Work out the finished part from the listing and answer in its coordinate system (mm). Face numbers are marked on the shaded views. A direction names the side the tool comes from. Round coordinates to 2 decimals unless told otherwise and drop trailing zeros. Loops run counter-clockwise (first coordinate to the right, second up) from the corner with the lowest first, then second, coordinate; pieces in that order, holes last. Notation, with made-up numbers: (75.5, 77.25) - (115.5, 77.25) arc R13 cw to (115.5, 99.25) - close; hole circle Ø2 at (58.25, 27.5). An arc over 180 degrees is marked (long way). Use CSV: the item, a comma, the result in double quotes. Start each with the question number.
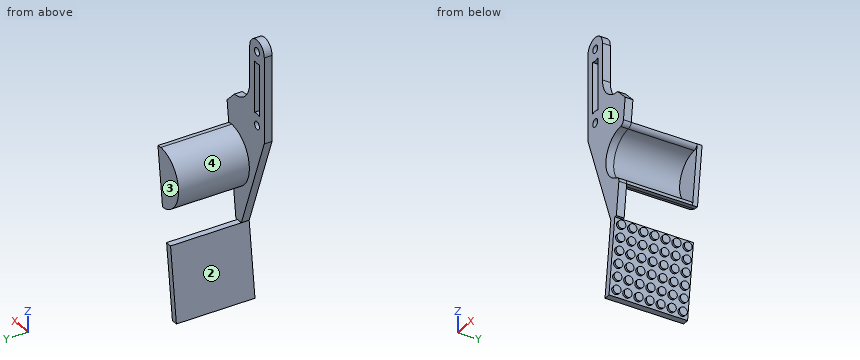
from build123d import *
from build123d.topology import SkipClean

# Parameters (mm, degrees)
CROQUIS1_R              = 1.5875
SALIENTE_EXTRUIR1_DEPTH = 3.175
CORTAR_EXTRUIR1_DEPTH   = 3.175
CORTAR_EXTRUIR3_DEPTH   = 10
CROQUIS4_R              = 10
CORTAR_EXTRUIR4_DEPTH   = 10
REDONDEO1_R             = 2
BOSS_EXTRUDE1_DEPTH     = 26.82
BOSS_EXTRUDE2_DEPTH     = 2
BOSS_EXTRUDE3_DEPTH     = 31.995
SKETCH5_R               = 1.59
BOSS_EXTRUDE4_DEPTH     = 1


with BuildPart() as part:
    # Croquis1 → Saliente-Extruir1 (new body)
    with BuildSketch(Plane(origin=(0, 0, 0), x_dir=(1, 0, 0), z_dir=(0, 1, 0))):
        with BuildLine():
            Line((-12.5, 0), (-12.5, -40))
            Line((-12.5, -40), (-2.975, -40))
            Line((-2.975, -40), (-2.975, -20))
            ThreePointArc((-2.975, -20), (-0.046067812, -12.928932188), (7.025, -10))
            Line((7.025, -10), (12.5, -10))
            Line((12.5, -10), (12.5, 40))
            Line((12.5, 40), (2.5, 40))
            Line((2.5, 40), (-12.5, 0))
        make_face()
        with Locations(Location((-7.7375, -5, 0), (0, 0, 270))):
            Circle(CROQUIS1_R, mode=Mode.SUBTRACT)
        with Locations(Location((-7.7375, -35, 0), (0, 0, 270))):
            Circle(CROQUIS1_R, mode=Mode.SUBTRACT)
    extrude(amount=SALIENTE_EXTRUIR1_DEPTH)

    # Croquis2 → Cortar-Extruir1 (cut)
    with BuildSketch(Plane(origin=(0, 3.175, 0), x_dir=(1, 0, 0), z_dir=(0, 1, 0))):
        Polygon((12.5, -10), (6.1, 40), (12.5, 40), align=None)
    extrude(amount=-CORTAR_EXTRUIR1_DEPTH, mode=Mode.SUBTRACT)

    # Croquis3 → Cortar-Extruir3 (cut)
    with BuildSketch(Plane(origin=(0, 3.175, 0), x_dir=(1, 0, 0), z_dir=(0, 1, 0))):
        with BuildLine():
            ThreePointArc((-5.975, -30.575635639), (-7.7375, -30.2375), (-9.5, -30.575635639))
            Line((-9.5, -30.575635639), (-9.5, -9.427055314))
            ThreePointArc((-9.5, -9.427055314), (-7.7375, -9.765), (-5.975, -9.427055314))
            Line((-5.975, -9.427055314), (-5.975, -14.803847577))
            Line((-5.975, -14.803847577), (-5.975, -30.575635639))
        make_face()
        with BuildLine():
            ThreePointArc((-12.5, -35), (-7.7375, -39.7625), (-2.975, -35))
            Line((-2.975, -35), (-2.975, -40))
            Line((-2.975, -40), (-12.5, -40))
            Line((-12.5, -40), (-12.5, -35))
        make_face()
    extrude(amount=-CORTAR_EXTRUIR3_DEPTH, mode=Mode.SUBTRACT)

    # Croquis4 → Cortar-Extruir4 (cut)
    with BuildSketch(Plane(origin=(0, 3.175, 0), x_dir=(1, 0, 0), z_dir=(0, 1, 0))):
        with Locations((9.274103387, 15.202317292)):
            Circle(CROQUIS4_R)
        Polygon((7.025, -10), (11.878723404, -5.146276596), (12.5, -10), align=None)
    extrude(amount=-CORTAR_EXTRUIR4_DEPTH, mode=Mode.SUBTRACT)

    # Redondeo1
    redondeo1_edges = [part.edges().sort_by_distance(p)[0] for p in [
        (8.004462032, 1.5875, -25.121390375),
        (10.543744741, 1.5875, -5.283244209),
    ]]
    fillet(redondeo1_edges, radius=REDONDEO1_R)

    # Sketch1 → Boss-Extrude1 (add)
    with SkipClean():  # the faces are left unmerged after this step: merging them gives an invalid solid
        with BuildSketch(Plane(origin=(0, 3.175, 0), x_dir=(1, 0, 0), z_dir=(0, 1, 0))):
            with BuildLine():
                Line((7.771843477, 26.938722839), (5.78802886, 26.684794568))
                ThreePointArc((5.78802886, 26.684794568), (-2.628784313, 13.678747666), (8.79254868, 3.211983474))
                Line((8.79254868, 3.211983474), (10.776363297, 3.465911745))
                ThreePointArc((10.776363297, 3.465911745), (10.143802127, 4.686471223), (8.872807798, 5.210372444))
                ThreePointArc((8.872807798, 5.210372444), (-0.644969697, 13.932675937), (6.369041281, 24.771048355))
                ThreePointArc((6.369041281, 24.771048355), (7.467102295, 25.59818866), (7.771843477, 26.938722839))
            make_face()
        extrude(amount=BOSS_EXTRUDE1_DEPTH)

    # Sketch2 → Boss-Extrude2 (add)
    with SkipClean():  # the faces are left unmerged after this step: merging them gives an invalid solid
        with BuildSketch(Plane(origin=(0, 29.995, 0), x_dir=(1, 0, 0), z_dir=(0, 1, 0))):
            with BuildLine():
                Line((10.776363297, 3.465911745), (7.771843477, 26.938722839))
                Line((7.771843477, 26.938722839), (5.78802886, 26.684794568))
                ThreePointArc((5.78802886, 26.684794568), (-2.628784313, 13.678747666), (8.79254868, 3.211983474))
                Line((8.79254868, 3.211983474), (10.776363297, 3.465911745))
            make_face()
        extrude(amount=BOSS_EXTRUDE2_DEPTH)

    # Sketch4 → Boss-Extrude3 (add)
    with SkipClean():  # the faces are left unmerged after this step: merging them gives an invalid solid
        with BuildSketch(Plane.XZ):
            Polygon((1.291075936, -69.75721925), (-1.308924064, -69.75721925), (2.5, -40), (5.1, -40), align=None)
        extrude(amount=-BOSS_EXTRUDE3_DEPTH)

    # Sketch5 → Boss-Extrude4 (add)
    with SkipClean():  # the faces are left unmerged after this step: merging them gives an invalid solid
        with BuildSketch(Plane(origin=(10.055254707, 0, -1.287072602), x_dir=(-0.12696413546540494, 0, -0.9919073083234755), z_dir=(0.9919073083234755, 0, -0.12696413546540494))):
            with Locations((41.528775242, 29.495)):
                Circle(SKETCH5_R)
            with Locations((46.528775242, 29.495)):
                Circle(SKETCH5_R)
            with Locations((51.528775242, 29.495)):
                Circle(SKETCH5_R)
            with Locations((56.528775242, 29.495)):
                Circle(SKETCH5_R)
            with Locations((61.528775242, 29.495)):
                Circle(SKETCH5_R)
            with Locations((66.528775242, 29.495)):
                Circle(SKETCH5_R)
            with Locations((46.528775242, 24.995)):
                Circle(SKETCH5_R)
            with Locations((51.528775242, 24.995)):
                Circle(SKETCH5_R)
            with Locations((56.528775242, 24.995)):
                Circle(SKETCH5_R)
            with Locations((61.528775242, 24.995)):
                Circle(SKETCH5_R)
            with Locations((66.528775242, 24.995)):
                Circle(SKETCH5_R)
            with Locations((46.528775242, 20.495)):
                Circle(SKETCH5_R)
            with Locations((51.528775242, 20.495)):
                Circle(SKETCH5_R)
            with Locations((56.528775242, 20.495)):
                Circle(SKETCH5_R)
            with Locations((61.528775242, 20.495)):
                Circle(SKETCH5_R)
            with Locations((66.528775242, 20.495)):
                Circle(SKETCH5_R)
            with Locations((46.528775242, 15.995)):
                Circle(SKETCH5_R)
            with Locations((51.528775242, 15.995)):
                Circle(SKETCH5_R)
            with Locations((56.528775242, 15.995)):
                Circle(SKETCH5_R)
            with Locations((61.528775242, 15.995)):
                Circle(SKETCH5_R)
            with Locations((66.528775242, 15.995)):
                Circle(SKETCH5_R)
            with Locations((46.528775242, 11.495)):
                Circle(SKETCH5_R)
            with Locations((51.528775242, 11.495)):
                Circle(SKETCH5_R)
            with Locations((56.528775242, 11.495)):
                Circle(SKETCH5_R)
            with Locations((61.528775242, 11.495)):
                Circle(SKETCH5_R)
            with Locations((66.528775242, 11.495)):
                Circle(SKETCH5_R)
            with Locations((46.528775242, 6.995)):
                Circle(SKETCH5_R)
            with Locations((51.528775242, 6.995)):
                Circle(SKETCH5_R)
            with Locations((56.528775242, 6.995)):
                Circle(SKETCH5_R)
            with Locations((61.528775242, 6.995)):
                Circle(SKETCH5_R)
            with Locations((66.528775242, 6.995)):
                Circle(SKETCH5_R)
            with Locations((46.528775242, 2.495)):
                Circle(SKETCH5_R)
            with Locations((51.528775242, 2.495)):
                Circle(SKETCH5_R)
            with Locations((56.528775242, 2.495)):
                Circle(SKETCH5_R)
            with Locations((61.528775242, 2.495)):
                Circle(SKETCH5_R)
            with Locations((66.528775242, 2.495)):
                Circle(SKETCH5_R)
            with Locations((41.528775242, 24.995)):
                Circle(SKETCH5_R)
            with Locations((41.528775242, 20.495)):
                Circle(SKETCH5_R)
            with Locations((41.528775242, 15.995)):
                Circle(SKETCH5_R)
            with Locations((41.528775242, 11.495)):
                Circle(SKETCH5_R)
            with Locations((41.528775242, 6.995)):
                Circle(SKETCH5_R)
            with Locations((41.528775242, 2.495)):
                Circle(SKETCH5_R)
        extrude(amount=BOSS_EXTRUDE4_DEPTH)


solid = part.part
Item 1: A cutting plane is placed at B-B (z = -10). Determine the outline of the cut face in (x, y) (3 decimals).
Item 2: The mould has two halves that part along Z. Classify the marked faces 3 and 4: pulls with the +Z half, pulls with the -Z half, needs draft (parallel to the pull), parting line crosses it, or undercut.
Item 3: Find the intervals of material crossed by probe 1 along Z at (x, y) = (3, 24.5); probe 2 along X at (y, z) = (1.1, 5) (3 decimals); probe 3 along X at (y, z) = (1.75, 35) (3 decimals), in increasing order. Write a range as [from, to].
Item 4: Each of these flat-tipped pins is pushed along its axis until it touches: pin 1 Ø3 at (x, y) = (4.5, 16.5) entering from +Z; pin 2 Ø4 at (x, z) = (-7.74, 5) entering from +Y (3 decimals); pin 3 Ø3.5 at (x, z) = (-7.74, 35) entering from -Y; pin 4 Ø3.5 at (y, z) = (1, 20) entering from +X. Where does it stop, or does it pass through?
Item 5: Which of the six approach directions +Z, -Z, +X, -X, +Y, -Y give full straight-line access (tool end or side, diameter ignored) to the marked faces 1 and 2?
Item 6: A cutting plane is placed at A-A (z = 27.5). Determine the outline of the cut face in (x, y) (3 decimals), plus the area to 4 significant figures.
Item 7: A cutting plane is placed at C-C (x = -11). Determine the outline of the cut face in (y, z) (3 decimals).
Item 8: A cutting plane is placed at D-D (z = -29.5). Determine the outline of the cut face in (x, y) (1 decimal), plus the area to 3 significant figures.
Result sheet:
1,outline,"(-8.75, 0) - (0.734, 0) - (0.734, 29.995) - (9.94, 29.995) - (9.94, 31.995) - (-1.54, 31.995) - (-1.54, 3.175) - (-8.75, 3.175) - close"
2,face 3,"needs draft"
2,face 4,"undercut"
3,probe 1,"[-63.94, -60.89], [-58.9, -40], [-25.43, -22.99], [-7.42, -4.97]"
3,probe 2,"[-12.5, -9.325], [-6.15, 11.86]"
3,probe 3,"[-12.5, -9.325], [-6.15, -2.975]"
4,pin 1,"z = -3.66"
4,pin 2,"y = 3.175"
4,pin 3,"y = 0"
4,pin 4,"x = -2.82"
5,face 1,"+Z, -Z, +X, -X, -Y"
5,face 2,"-X, +Y, -Y"
6,outline,"(-12.5, 0) - (-9.5, 0) - (-9.5, 3.175) - (-12.5, 3.175) - close; (-5.975, 0) - (-2.975, 0) - (-2.975, 3.175) - (-5.975, 3.175) - close"
6,area,"19.05 mm^2"
7,outline,"(0, -4) - (3.175, -4) - (3.175, 38.47) - (0, 38.47) - close"
8,outline,"(-1.4, 0) - (7.4, 0) - (7.4, 3.2) - (-1.4, 3.2) - close"
8,area,"28.2 mm^2"
